Here's the drawing with two shaded views (mm, measured from the low corner). I have some questions. Round coordinates to 2 decimals unless told otherwise and drop trailing zeros. Write each loop counter-clockwise with the first axis right and the second up, starting at its lowest first coordinate (ties: lowest second). Pieces come first, ordered by that corner, then holes. Notation, with made-up numbers: M 88.5,34.5 L 113.5,34.5 A22 ccw 113.5,56.5 Z; hole C 26.5,26.5 d10. An arc over 180 degrees is marked long. Write item = value, one per line. Start each with the question number.
(1) I want a section at C-C (y = 5). List the corners of the cut face in (x, z) for me, and give its area (3 significant figures).
(2) I want a section at D-D (x = 40.5). List the corners of the cut face in (y, z) for me (1 decimal), and give its area (3 significant figures).
(3) I need wall thicknesses on line 1 along Y through (x, z) = (24, 3) (1 decimal). Which ranges of the line are inside material? Lowest first, please.
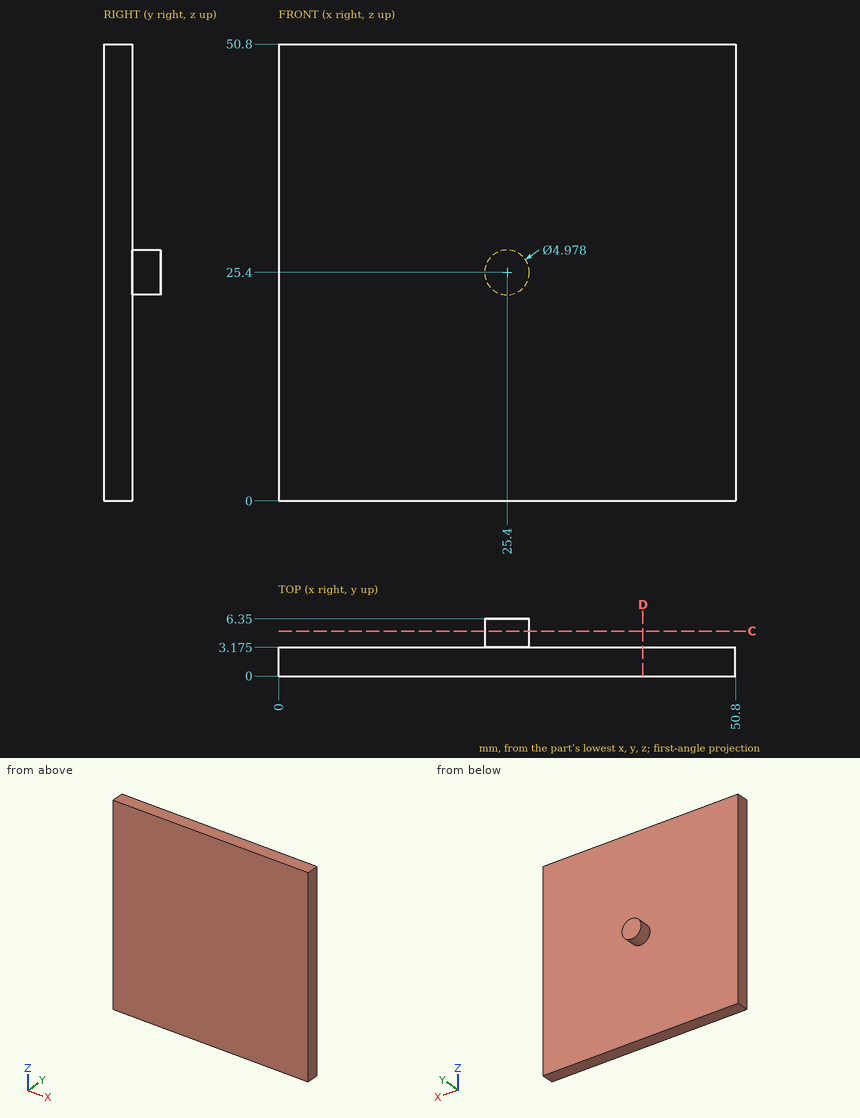
Returned:
q1.outline = C 25.4,25.4 d4.98
q1.area = 19.5 mm²
q2.outline = M 0,0 L 3.2,0 L 3.2,50.8 L 0,50.8 Z
q2.area = 161 mm²
q3.line_1 = 0 to 3.2
